Can you work these out from the model? Positions are in its coordinate system, mm. A direction names the side the tool comes from. Round coordinates to 2 decimals unless told otherwise and drop trailing zeros. Loops run counter-clockwise (first coordinate to the right, second up) from the corner with the lowest first, then second, coordinate; pieces in that order, holes last. Notation, with made-up numbers: M 56,3 L 96,3 A16 cw 96,33 Z; hole C -13,55.25 d11. An arc over 180 degrees is marked long. Use a Markdown table: item, result. Add a question column.
```python
from build123d import *

# Parameters (mm, degrees)
SKETCH2_R           = 25
SKETCH2_R_2         = 15
BOSS_EXTRUDE1_DEPTH = 200
SKETCH5_R           = 7.5
BOSS_EXTRUDE2_DEPTH = 25


with BuildPart() as part:
    # Sketch2 → Boss-Extrude1 (new body)
    with BuildSketch(Plane(origin=(0, 0, 0), x_dir=(1, 0, 0), z_dir=(0, 1, 0))):
        Circle(SKETCH2_R)
        Circle(SKETCH2_R_2, mode=Mode.SUBTRACT)
    extrude(amount=BOSS_EXTRUDE1_DEPTH)

    # Sketch5 → Boss-Extrude2 (add, symmetric)
    with BuildSketch(Plane(origin=(0, 0, 0), x_dir=(0, -1, 0), z_dir=(-1, 0, 0))):
        with BuildLine():
            Line((0, 29.012112286), (9.706174679, 29.012112286))
            ThreePointArc((9.706174679, 29.012112286), (38.670140077, 0.993968953), (11.62868774, -28.883907525))
            Line((11.62868774, -28.883907525), (0, -28.883907525))
            Line((0, -28.883907525), (0, 29.012112286))
        make_face()
        with Locations((9.706174679, 0)):
            Circle(SKETCH5_R, mode=Mode.SUBTRACT)
    extrude(amount=BOSS_EXTRUDE2_DEPTH, both=True)


solid = part.part
```
(1) Thinking about a two-plate mould opening in Z: for faces 1 (the face through (0, -6, -28.884)), 2 (the face through (0.35, -16.634, -2.873)), 3 (the face through (23.846, 98.6, -7.509)), which applies, released by +Z, released by -Z, zero draft, split by the parting line, or undercut?
(2) On a 3-axis mill with a long thin cutter (end or side, diameter ignored), from which of +Z, -Z, +X, -X, +Y, -Y can I reach the whole of each face in a straight line? I mean faces 4 (the face through (-0.1, 0, 25.2)), 5 (the face through (-25, -20, 0)), 6 (the face through (0, 0, 0)), 7 (the face through (0, -5, 29.012)), 8 (the face through (-4, 0, -25)). Say none if no direction works.
(3) I'm going to push flat-ended pins straight in: pin 1 (1.5 mm diameter, centred on y = 116, z = -14, fed in from -X); pin 2 (12 mm diameter, centred on x = -20, y = 84.5, fed in from -Z); pin 3 (6 mm diameter, centred on y = 81.5, z = 18.5, fed in from +X). Where does each tip first touch, or does it pass through?
(4) Suppose I cut it at C-C on y = 37.5. List the corners of the cut face in (x, z) for me.
(5) Suppose I cut it at A-A on x = 0. List the corners of the cut face in (y, z) for me, and give its area (3 significant figures).
(6) If I drill on probe 1 along Z at (x, y) = (0, 50.5); probe 2 along Y at (x, z) = (-8.5, -4.5), over which ranges is the centre line in solid material (lowest first)? Write a range as [from, to].
(7) Suppose I cut it at D-D on x = 20. List the corners of the cut face in (y, z) for me, and give its area (3 significant figures).
(8) Suppose I cut it at B-B on z = 20.5. List the corners of the cut face in (x, y) for me.
Results below:
| question | item | result |
|---|---|---|
| 1 | face 1 | released by -Z |
| 1 | face 2 | undercut |
| 1 | face 3 | split by the parting line |
| 2 | face 4 | +Z, +Y |
| 2 | face 5 | +Z, -Z, -X, +Y, -Y |
| 2 | face 6 | +Y |
| 2 | face 7 | +Z, +X, -X, +Y, -Y |
| 2 | face 8 | -Z, +Y |
| 3 | pin 1 | stops at x = -21.2 |
| 3 | pin 2 | stops at z = -20.71 |
| 3 | pin 3 | stops at x = 19.62 |
| 4 | outline | C 0,0 d50; hole C 0,0 d30 |
| 5 | outline | M -11.63,-28.88 L 0,-28.88 L 0,-25 L 200,-25 L 200,-15 L 0,-15 L 0,15 L 200,15 L 200,25 L 0,25 L 0,29.01 L -9.71,29.01 A28.98 ccw Z; hole C -9.71,0 d15 |
| 5 | area | 5,700 mm² |
| 6 | probe 1 | z = [-25, -15], [15, 25] |
| 6 | probe 2 | y = [-38.33, -15.71], [-3.71, 0] |
| 7 | outline | M -11.63,-28.88 L 0,-28.88 L 0,-15 L 200,-15 L 200,15 L 0,15 L 0,29.01 L -9.71,29.01 A28.98 ccw Z; hole C -9.71,0 d15 |
| 7 | area | 7,700 mm² |
| 8 | outline | M -25,-30.22 L 25,-30.22 L 25,0 L 14.31,0 L 14.31,200 L -14.31,200 L -14.31,0 L -25,0 Z |
